from build123d import *

# Parameters (mm, degrees)
F1_DEPTH = 12.7
F2_DEPTH = 7.62


with BuildPart() as f1:
    # F0 (on Right) → F1 (new body, symmetric)
    with BuildSketch(Plane.YZ):
        with BuildLine():
            Line((19.05, 2.192055), (6.210823, 6.35))
            Line((6.210823, 6.35), (-19.05, 6.35))
            ThreePointArc((-19.05, 6.35), (-14.559872, 4.490128), (-12.7, 0))
            ThreePointArc((-12.7, 0), (-14.559872, -4.490128), (-19.05, -6.35))
            Line((-19.05, -6.35), (10.473152, -6.35))
            Line((10.473152, -6.35), (19.05, -6.35))
            Line((19.05, -6.35), (19.05, 2.192055))
        make_face()
    extrude(amount=F1_DEPTH, both=True)

    # F0 (on Right) → F2 (join, symmetric)
    with BuildSketch(Plane.YZ):
        with BuildLine():
            ThreePointArc((-12.7, 0), (-14.559872, 4.490128), (-19.05, 6.35))
            Line((-19.05, 6.35), (-19.05, -6.35))
            ThreePointArc((-19.05, -6.35), (-14.559872, -4.490128), (-12.7, 0))
        make_face()
        with BuildLine():
            Line((-19.05, -6.35), (-19.05, 6.35))
            ThreePointArc((-19.05, 6.35), (-25.4, 0), (-19.05, -6.35))
        make_face()
    extrude(amount=F2_DEPTH, both=True)


solid = f1.part
Model file for the job. Use its own axes, mm. A direction names the side the tool comes from. Give positions to 0.01 mm unless a question says otherwise; leave off trailing zeros. Loops run counter-clockwise (first coordinate to the right, second up) from the corner with the lowest first, then second, coordinate; pieces in that order, holes last. Notation, with made-up numbers: (77.25, 73.25) -> (101.25, 73.25) arc R21 ccw to (101.25, 106.25) -> close; hole circle Ø6 at (-38.5, 31.25). An arc over 180 degrees is marked (long way). Use a Markdown table: item, result. Add a question column.
(1) Wall check: line 1 along X through (y, z) = (-19.5, 3); line 2 along Y through (x, z) = (4, -0.25); line 3 along Z through (x, y) = (-5.75, 10). Give the ranges that are in metal, low to high.
(2) Drop flat-ended pins along their axis: pin 1 Ø4 at (y, z) = (-16.5, 3) entering from -X; pin 2 Ø3 at (x, y) = (8.5, 10.5) entering from +Z; pin 3 Ø2 at (x, y) = (1.5, 12.5) entering from +Z. Give the stop position or say it passes through.
(3) Slice it at D-D on z = -0.75. List the corners of the cut face in (x, y), and give its area (4 significant figures).
(4) Tool access for faces 1 (the flat face through (7.62, -19, 0)), 2 (the flat face through (-7.62, -19, 0)), 3 (the flat face through (0, 19.05, -2)): list every direction of +Z, -Z, +X, -X, +Y, -Y with a clear straight run to the whole face (end or side of a thin tool).
(5) Slice it at C-C on y = -14. List the corners of the cut face in (x, z), and give its area (3 significant figures).
(6) Slice it at B-B on z = 1.5. List the corners of the cut face in (x, y), and give its area (3 significant figures).
(7) Slice it at A-A on x = 10. List the corners of the cut face in (y, z), and give its area (3 significant figures).
Filled sheet:
| question | item | result |
|---|---|---|
| 1 | line 1 | -7.62 to 7.62 |
| 1 | line 2 | -25.4 to 19.05 |
| 1 | line 3 | -6.35 to 5.12 |
| 2 | pin 1 | x = -7.62 |
| 2 | pin 2 | z = 5.45 |
| 2 | pin 3 | z = 4.64 |
| 3 | outline | (-12.7, -12.74) -> (-7.62, -12.74) -> (-7.62, -25.36) -> (7.62, -25.36) -> (7.62, -12.74) -> (12.7, -12.74) -> (12.7, 19.05) -> (-12.7, 19.05) -> close |
| 3 | area | 1,000 mm2 |
| 4 | face 1 | +X, -Y |
| 4 | face 2 | -X, -Y |
| 4 | face 3 | +Z, -Z, +X, -X, +Y |
| 5 | outline | (-12.7, -6.35) -> (12.7, -6.35) -> (12.7, -3.85) -> (7.62, -3.85) -> (7.62, 3.85) -> (12.7, 3.85) -> (12.7, 6.35) -> (-12.7, 6.35) -> (-12.7, 3.85) -> (-7.62, 3.85) -> (-7.62, -3.85) -> (-12.7, -3.85) -> close |
| 5 | area | 244 mm2 |
| 6 | outline | (-12.7, -12.88) -> (-7.62, -12.88) -> (-7.62, -25.22) -> (7.62, -25.22) -> (7.62, -12.88) -> (12.7, -12.88) -> (12.7, 19.05) -> (-12.7, 19.05) -> close |
| 6 | area | 999 mm2 |
| 7 | outline | (-19.05, -6.35) -> (19.05, -6.35) -> (19.05, 2.19) -> (6.21, 6.35) -> (-19.05, 6.35) arc R6.35 cw to start |
| 7 | area | 394 mm2 |
